Could you check a few things on this model? Use its own coordinates, in mm. A direction names the side the tool comes from. Coordinates: 2 decimals unless noted, no trailing zeros. Loops run counter-clockwise (first coordinate to the right, second up) from the corner with the lowest first, then second, coordinate; pieces in that order, holes last. Notation, with made-up numbers: M 79.25,25.5 L 95.25,25.5 A24 cw 95.25,59.5 Z; hole C 6.25,-27.75 d5. An arc over 180 degrees is marked long. Return JSON: item names as keys, results as strings. Group by question number.
from build123d import *

# Parameters (mm, degrees)
SKETCH2_W           = 139.7
SKETCH2_H           = 139.7
BOSS_EXTRUDE1_DEPTH = 10
SKETCH1_R           = 3.5
CUT_EXTRUDE1_DEPTH  = 10
SKETCH3_W           = 21.5
SKETCH3_H           = 31
CUT_EXTRUDE2_DEPTH  = 1.6
SKETCH4_R           = 1.7
CUT_EXTRUDE3_DEPTH  = 10
CUT_EXTRUDE4_DEPTH  = 2


with BuildPart() as part:
    # Sketch2 → Boss-Extrude1 (new body)
    with BuildSketch(Plane(origin=(0, 0, 0), x_dir=(1, 0, 0), z_dir=(0, 1, 0))):
        with Locations((69.85, 69.85)):
            Rectangle(SKETCH2_W, SKETCH2_H)
    extrude(amount=BOSS_EXTRUDE1_DEPTH)

    # Sketch1 → Cut-Extrude1 (cut)
    with BuildSketch(Plane(origin=(0, 10, 0), x_dir=(1, 0, 0), z_dir=(0, 1, 0))):
        with BuildLine():
            Line((6.35, 136.85), (6.35, 133.35))
            Line((6.35, 133.35), (2.85, 133.35))
            ThreePointArc((2.85, 133.35), (6.35, 129.85), (9.85, 133.35))
            ThreePointArc((9.85, 133.35), (8.824873734, 135.824873734), (6.35, 136.85))
        make_face()
        with BuildLine():
            Line((2.85, 133.35), (6.35, 133.35))
            Line((6.35, 133.35), (6.35, 136.85))
            ThreePointArc((6.35, 136.85), (3.875126266, 135.824873734), (2.85, 133.35))
        make_face()
        with Locations((133.35, 133.35)):
            Circle(SKETCH1_R)
        with Locations((6.35, 6.35)):
            Circle(SKETCH1_R)
        with Locations((133.35, 6.35)):
            Circle(SKETCH1_R)
    extrude(amount=-CUT_EXTRUDE1_DEPTH, mode=Mode.SUBTRACT)

    # Sketch3 → Cut-Extrude2 (cut)
    with BuildSketch(Plane(origin=(0, 10, 0), x_dir=(1, 0, 0), z_dir=(0, 1, 0))):
        with Locations((71.85, 58.1468)):
            Rectangle(SKETCH3_W, SKETCH3_H)
    extrude(amount=-CUT_EXTRUDE2_DEPTH, mode=Mode.SUBTRACT)

    # Sketch4 → Cut-Extrude3 (cut)
    with BuildSketch(Plane(origin=(0, 10, 0), x_dir=(1, 0, 0), z_dir=(0, 1, 0))):
        with Locations((7.85, 114.1468)):
            Circle(SKETCH4_R)
        with Locations((7.85, 18.1468)):
            Circle(SKETCH4_R)
        with Locations((117.85, 114.1468)):
            Circle(SKETCH4_R)
        with Locations((117.85, 18.1468)):
            Circle(SKETCH4_R)
    extrude(amount=-CUT_EXTRUDE3_DEPTH, mode=Mode.SUBTRACT)

    # Sketch5 → Cut-Extrude4 (cut)
    with BuildSketch(Plane(origin=(0, 10, 0), x_dir=(1, 0, 0), z_dir=(0, 1, 0))):
        Polygon((9.582050808, 111.1468), (11.314101615, 114.1468), (9.582050808, 117.1468), (6.117949192, 117.1468), (4.385898385, 114.1468), (6.117949192, 111.1468), align=None)
        Polygon((9.582050808, 15.1468), (11.314101615, 18.1468), (9.582050808, 21.1468), (6.117949192, 21.1468), (4.385898385, 18.1468), (6.117949192, 15.1468), align=None)
        Polygon((119.582050808, 111.1468), (121.314101615, 114.1468), (119.582050808, 117.1468), (116.117949192, 117.1468), (114.385898385, 114.1468), (116.117949192, 111.1468), align=None)
        Polygon((119.582050808, 15.1468), (121.314101615, 18.1468), (119.582050808, 21.1468), (116.117949192, 21.1468), (114.385898385, 18.1468), (116.117949192, 15.1468), align=None)
    extrude(amount=-CUT_EXTRUDE4_DEPTH, mode=Mode.SUBTRACT)


solid = part.part
(1) Imagine slicing it at C-C, the plane z = -48. Write out the boundary of the cut face in (x, y), then the cut area to 3 significant figures.
(2) We'd pull the mould along Z, two halves only. Please class faces 1 (the face through (119.42, 4.06, -17.5)), 2 (the face through (69, 5, -139.7)), 3 (the face through (69, 0, -71)): +Z half, -Z half, draft (parallel to the pull), parting line (faces both ways), or undercut.
(3) If I drill on L1, parallel to Z at x = 133.35, y = 6; L2, parallel to X at y = 6.75, z = -6.35; L3, parallel to X at y = 9, z = -47.5, over which ranges is the centre line in solid material (lowest first)? Write a range as [from, to].
(4) Imagine slicing it at A-A, the plane z = -6.35. Write out the boundary of the cut face in (x, y), then the cut area to 3 significant figures.
(5) Will these pins go through, and if not, where does the flat tip stop? P1, Ø3, axis at x = 6.5, z = -114.5, coming from the +Y side; P2, Ø1, axis at x = 8.5, y = 9, coming from the +Z side; P3, Ø2.5, axis at x = 117.85, z = -114.15, coming from the -Y side; P4, Ø17, axis at x = 70.5, z = -52, coming from the +Y side.
(6) Imagine slicing it at B-B, the plane x = 117.85. Write out the boundary of the cut face in (y, z), then the cut area to 3 significant figures.
(7) For faces 4 (the face through (119.47, 4.06, -114.66)), 5 (the face through (72, 8.4, -58)), which set-ups out of +Z, -Z, +X, -X, +Y, -Y let a thin tool reach every point of the face, with its end or its side?
Checks:
{
 "1": {"outline": "M 0,0 L 139.7,0 L 139.7,10 L 82.6,10 L 82.6,8.4 L 61.1,8.4 L 61.1,10 L 0,10 Z", "area": "1,360 mm²"},
 "2": {"face 1": "undercut", "face 2": "-Z half", "face 3": "draft"},
 "3": {"L1": "[-139.7, -136.85], [-129.85, -9.85], [-2.85, 0]", "L2": "[0, 2.85], [9.85, 129.85], [136.85, 139.7]", "L3": "[0, 61.1], [82.6, 139.7]"},
 "4": {"outline": "M 0,0 L 2.85,0 L 2.85,10 L 0,10 Z; M 9.85,0 L 129.85,0 L 129.85,10 L 9.85,10 Z; M 136.85,0 L 139.7,0 L 139.7,10 L 136.85,10 Z", "area": "1,260 mm²"},
 "5": {"P1": "y = 8", "P2": "z = 0", "P3": "through", "P4": "y = 8.4"},
 "6": {"outline": "M 0,-139.7 L 10,-139.7 L 10,-117.15 L 8,-117.15 L 8,-115.85 L 0,-115.85 Z; M 0,-112.45 L 8,-112.45 L 8,-111.15 L 10,-111.15 L 10,-21.15 L 8,-21.15 L 8,-19.85 L 0,-19.85 Z; M 0,-16.45 L 8,-16.45 L 8,-15.15 L 10,-15.15 L 10,0 L 0,0 Z", "area": "1,320 mm²"},
 "7": {"face 4": "+Y, -Y", "face 5": "+Y"}
}
